```python
from build123d import *

# Parameters (mm, degrees)
SKETCH1_W           = 160
SKETCH1_H           = 300
BOSS_EXTRUDE1_DEPTH = 3
SKETCH1_3_W         = 30
SKETCH1_3_H         = 13
BOSS_EXTRUDE2_DEPTH = 4


with BuildPart() as part:
    # Sketch1 → Boss-Extrude1 (new body)
    with BuildSketch(Plane(origin=(0, 0, 0), x_dir=(1, 0, 0), z_dir=(0, 1, 0))):
        with Locations((120.485764952, -89.40841277)):
            Rectangle(SKETCH1_W, SKETCH1_H)
        Polygon((50.485764952, -44.40841277), (50.485764952, 30.59158723), (75.485764952, 30.59158723), (75.485764952, -0.40841277), (105.485764952, -0.40841277), (105.485764952, -13.40841277), (75.485764952, -13.40841277), (75.485764952, -44.40841277), align=None, mode=Mode.SUBTRACT)
        Polygon((165.485764952, -0.40841277), (165.485764952, 30.59158723), (190.485764952, 30.59158723), (190.485764952, -44.40841277), (165.485764952, -44.40841277), (165.485764952, -13.40841277), (135.485764952, -13.40841277), (135.485764952, -0.40841277), align=None, mode=Mode.SUBTRACT)
    extrude(amount=BOSS_EXTRUDE1_DEPTH)

    # Sketch1<3> → Boss-Extrude2 (add)
    with BuildSketch(Plane(origin=(0, 0, 0), x_dir=(1, 0, 0), z_dir=(0, 1, 0))):
        with Locations((90.485764952, -6.90841277)):
            Rectangle(SKETCH1_3_W, SKETCH1_3_H)
        with Locations((150.485764952, -6.90841277)):
            Rectangle(SKETCH1_3_W, SKETCH1_3_H)
    extrude(amount=BOSS_EXTRUDE2_DEPTH)


solid = part.part
```
Here's how the part is built. I have some questions about the finished solid (model axes, mm). Round coordinates to 2 decimals unless told otherwise and drop trailing zeros. Order: outer loops, then holes, each group sorted by start corner. A loop starts at its lowest first (then second) coordinate and runs counter-clockwise, first axis right, second up. Notation, with made-up numbers: M 67,-22 L 74,-22 A11 ccw 74,-2 Z; hole C 51.25,72.5 d4. An arc over 180 degrees is marked long. Answer in a Markdown table with one row per item.
Item 1: Imagine slicing it at D-D, the plane x = 85.5. Write out the boundary of the cut face in (y, z), and give its area (3 significant figures).
A:
| item | result |
|---|---|
| outline | M 0,-60.59 L 3,-60.59 L 3,0.41 L 4,0.41 L 4,13.41 L 3,13.41 L 3,239.41 L 0,239.41 Z |
| area | 913 mm2 |
Item 2: Imagine slicing it at C-C, the plane y = 1.25. Write out the boundary of the cut face in (x, z).
A:
| item | result |
|---|---|
| outline | M 40.49,-60.59 L 200.49,-60.59 L 200.49,239.41 L 40.49,239.41 Z; hole M 50.49,-30.59 L 75.49,-30.59 L 75.49,44.41 L 50.49,44.41 Z; hole M 165.49,-30.59 L 190.49,-30.59 L 190.49,44.41 L 165.49,44.41 Z |
Item 3: Imagine slicing it at A-A, the plane x = 64. Write out the boundary of the cut face in (y, z), and give its area (3 significant figures).
A:
| item | result |
|---|---|
| outline | M 0,-60.59 L 3,-60.59 L 3,-30.59 L 0,-30.59 Z; M 0,44.41 L 3,44.41 L 3,239.41 L 0,239.41 Z |
| area | 675 mm2 |
Item 4: I'm going to push flat-ended pins straight in: pin 1 (0.8 mm diameter, centred on x = 92.5, y = 3.5, fed in from -Z); pin 2 (3 mm diameter, centred on x = 177, z = 144, fed in from +Y); pin 3 (0.5 mm diameter, centred on x = 85, y = 3.5, fed in from +Z). Where does each tip first touch, or does it pass through?
A:
| item | result |
|---|---|
| pin 1 | stops at z = 0.41 |
| pin 2 | stops at y = 3 |
| pin 3 | stops at z = 13.41 |
Item 5: If I drill on L1, parallel to X at y = 2.7, z = 24.5; L2, parallel to Z at x = 64.5, y = 1.55; L3, parallel to Y at x = 52, z = 96.5, over which ranges is the centre line in solid material (lowest first)? Write a range as from..to.
A:
| item | result |
|---|---|
| L1 | x = 40.49..50.49, 75.49..165.49, 190.49..200.49 |
| L2 | z = -60.59..-30.59, 44.41..239.41 |
| L3 | y = 0..3 |
Item 6: Imagine slicing it at B-B, the plane z = 39.5. Write out the boundary of the cut face in (x, y).
A:
| item | result |
|---|---|
| outline | M 40.49,0 L 50.49,0 L 50.49,3 L 40.49,3 Z; M 75.49,0 L 165.49,0 L 165.49,3 L 75.49,3 Z; M 190.49,0 L 200.49,0 L 200.49,3 L 190.49,3 Z |
